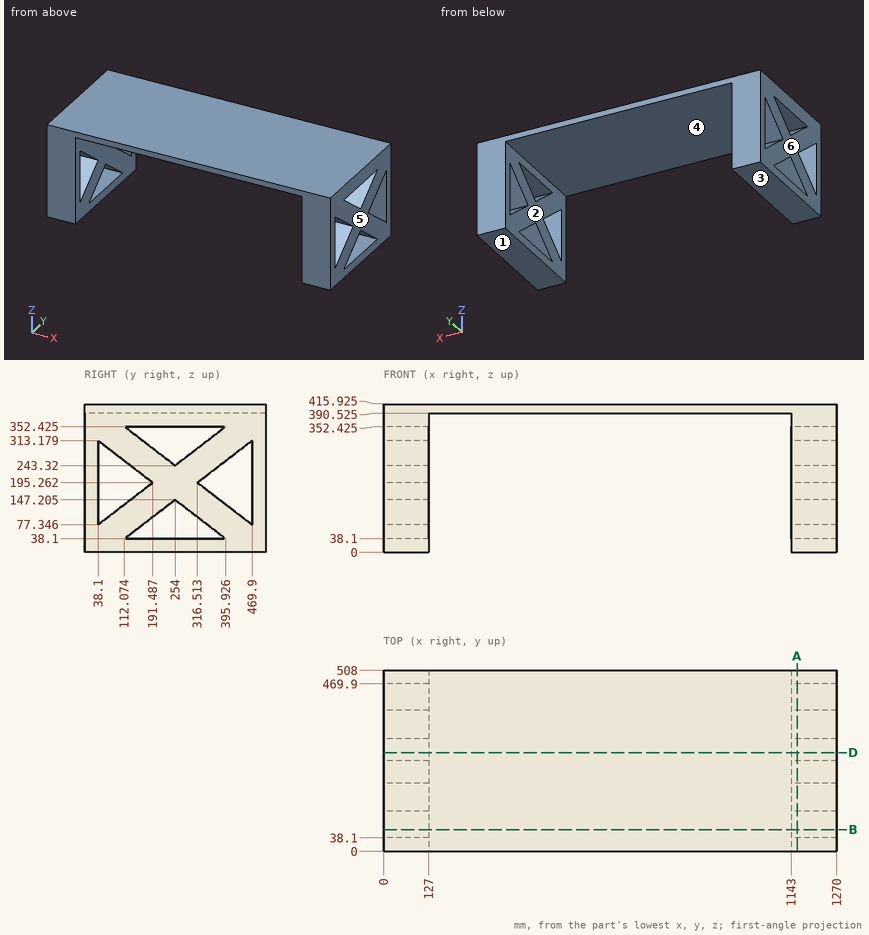
Check sheet for the drawn part. Datum: minimum x, y, z corner. Units: mm. A direction names the side the tool comes from. Give positions to 0.01 mm unless a question says otherwise; leave off trailing zeros. Order: outer loops, then holes, each group sorted by start corner. A loop starts at its lowest first (then second) coordinate and runs counter-clockwise, first axis right, second up. Notation, with made-up numbers: (58.25, -8.5) -> (71.25, -8.5) arc R9 cw to (71.25, -3.5) -> close; hole circle Ø5 at (48.5, -3.75). An arc over 180 degrees is marked (long way). Use a Markdown table: item, result.
1) Material ranges on probe 1 along X at (y, z) = (183.5, 141.5); probe 2 along Z at (x, y) = (521, 99.5) (1 decimal), recorded low to high.
Results:
| item | result |
|---|---|
| probe 1 | 0 to 127, 1143 to 1270 |
| probe 2 | 390.5 to 415.9 |
2) Section check D-D, the plane y = 277. Record the boundary of the cut face in (x, z) (1 decimal).
Results:
| item | result |
|---|---|
| outline | (0, 0) -> (127, 0) -> (127, 38.1) -> (0, 38.1) -> close; (0, 129.5) -> (127, 129.5) -> (127, 261) -> (0, 261) -> close; (0, 352.4) -> (127, 352.4) -> (127, 390.5) -> (1143, 390.5) -> (1143, 352.4) -> (1270, 352.4) -> (1270, 415.9) -> (0, 415.9) -> close; (1143, 0) -> (1270, 0) -> (1270, 38.1) -> (1143, 38.1) -> close; (1143, 129.5) -> (1270, 129.5) -> (1270, 261) -> (1143, 261) -> close |
3) Tool access check on the marked faces 1 and 2. Record the directions out of +Z, -Z, +X, -X, +Y, -Y that give a thin tool (end or side, any length) a straight path to the whole face; none if there is none.
Results:
| item | result |
|---|---|
| face 1 | -Z, +X, -X, +Y, -Y |
| face 2 | -Z, +Y, -Y |
4) Mould release check, pull along X, two halves, no side actions. Record for the marked faces 3, 4, 5 and 6: pulls with the +X half, pulls with the -X half, needs draft (parallel to the pull), parting line crosses it, or undercut.
Results:
| item | result |
|---|---|
| face 3 | needs draft |
| face 4 | undercut |
| face 5 | pulls with the +X half |
| face 6 | pulls with the -X half |
5) Depth check by flat-ended pin: pin 1 Ø12 at (x, y) = (751, 448.5) entering from -Z (1 decimal). Enter the tip coordinate at first touch or a pass-through.
Results:
| item | result |
|---|---|
| pin 1 | z = 390.5 |
6) Section check A-A, the plane x = 1159.5. Record the boundary of the cut face in (y, z) (1 decimal).
Results:
| item | result |
|---|---|
| outline | (0, 0) -> (508, 0) -> (508, 415.9) -> (0, 415.9) -> close; hole (38.1, 77.3) -> (191.5, 195.3) -> (38.1, 313.2) -> close; hole (112.1, 38.1) -> (395.9, 38.1) -> (254, 147.2) -> close; hole (112.1, 352.4) -> (254, 243.3) -> (395.9, 352.4) -> close; hole (316.5, 195.3) -> (469.9, 77.3) -> (469.9, 313.2) -> close |
7) Section check B-B, the plane y = 61. Give the number of separate pieces and of enclosed holes in the cut face, then the cut area to 3 significant figures.
Results:
| item | result |
|---|---|
| separate pieces | 3 |
| enclosed holes | 0 |
| area | 80,500 mm² |
